```python
from build123d import *

# Parameters (mm, degrees)
SKETCH1_W                 = 38
SKETCH1_H                 = 30
BOSS_EXTRUDE1_DEPTH       = 64.4
SKETCH3_R                 = 13
BOSS_EXTRUDE3_DEPTH       = 17
SKETCH2_R                 = 4
BOSS_EXTRUDE4_DEPTH       = 18.25
SKETCH16_W                = 32
SKETCH16_H                = 58.4
CUT_EXTRUDE1_DEPTH        = 90.955669638
SKETCH17_R                = 15
BOSS_EXTRUDE9_DEPTH       = 58.4
FILLET1_R                 = 1
M3X0_5_TAPPED_HOLE1_D     = 2.5
M3X0_5_TAPPED_HOLE1_DEPTH = 3
M3X0_5_TAPPED_HOLE2_D     = 2.5
M3X0_5_TAPPED_HOLE2_DEPTH = 3
SKETCH22_R                = 4
SKETCH22_R_2              = 2.5
CUT_EXTRUDE2_DEPTH        = 13.25
FILLET2_R                 = 0.5


with BuildPart() as part:
    # Sketch1 → Boss-Extrude1 (new body)
    with BuildSketch(Plane.XY):
        Rectangle(SKETCH1_W, SKETCH1_H)
    extrude(amount=BOSS_EXTRUDE1_DEPTH)

    # Sketch3 → Boss-Extrude3 (add)
    with BuildSketch(Plane(origin=(0, 0, 0), x_dir=(-1, 0, 0), z_dir=(0, 0, -1))):
        Circle(SKETCH3_R)
    extrude(amount=BOSS_EXTRUDE3_DEPTH)

    # Sketch2 → Boss-Extrude4 (add)
    with BuildSketch(Plane.XY.offset(64.4)):
        with Locations(Location((0, 0, 0), (0, 0, 180))):
            Circle(SKETCH2_R)
    extrude(amount=BOSS_EXTRUDE4_DEPTH)

    # Sketch16 → Cut-Extrude1 (cut, through all)
    with BuildSketch(Plane.XZ.offset(15)):
        with Locations((0, 32.2)):
            Rectangle(SKETCH16_W, SKETCH16_H)
    extrude(amount=-CUT_EXTRUDE1_DEPTH, mode=Mode.SUBTRACT)

    # Sketch17 → Boss-Extrude9 (add)
    with BuildSketch(Plane(origin=(0, 0, 61.4), x_dir=(-1, 0, 0), z_dir=(0, 0, -1))):
        with Locations(Location((0, 0, 0), (0, 0, 270))):
            Circle(SKETCH17_R)
    extrude(amount=BOSS_EXTRUDE9_DEPTH)

    # Fillet1
    fillet1_edges = [part.edges().sort_by_distance(p)[0] for p in [
        (-19, 0, 64.4),
        (19, 0, 64.4),
    ]]
    fillet(fillet1_edges, radius=FILLET1_R)

    # M3x0.5 Tapped Hole1
    with Locations(Plane.ZY.offset(19)):
        with Locations((14.4, -10), (44.4, -10), (44.4, 10), (14.4, 10)):
            Hole(M3X0_5_TAPPED_HOLE1_D / 2, depth=M3X0_5_TAPPED_HOLE1_DEPTH)

    # M3x0.5 Tapped Hole2
    with Locations(Plane(origin=(19, 0, 0), x_dir=(0, 0, -1), z_dir=(1, 0, 0))):
        with Locations((-14.4, 10), (-14.4, -10), (-44.4, -10), (-44.4, 10)):
            Hole(M3X0_5_TAPPED_HOLE2_D / 2, depth=M3X0_5_TAPPED_HOLE2_DEPTH)

    # Sketch22 → Cut-Extrude2 (cut)
    with BuildSketch(Plane.XY.offset(64.4)):
        Circle(SKETCH22_R)
        Circle(SKETCH22_R_2, mode=Mode.SUBTRACT)
    extrude(amount=CUT_EXTRUDE2_DEPTH, mode=Mode.SUBTRACT)

    # Fillet2
    fillet2_edges = [part.edges().sort_by_distance(p)[0] for p in [
        (4, 0, 82.65),
    ]]
    fillet(fillet2_edges, radius=FILLET2_R)


solid = part.part
```
Read the model definition and answer for the solid it produces. Units are mm, in the model's axes. A direction names the side the tool comes from. Give positions to 0.01 mm unless a question says otherwise; leave off trailing zeros. Write each loop counter-clockwise with the first axis right and the second up, starting at its lowest first coordinate (ties: lowest second). Pieces come first, ordered by that corner, then holes. Notation, with made-up numbers: (7.5, 44.25) - (61.5, 44.25) arc R14 cw to (61.5, 49.25) - close; hole circle Ø11 at (-15.75, 76.5). An arc over 180 degrees is marked (long way). Write item = value, one per line. Start each with the question number.
Item 1: Each of these flat-tipped pins is pushed along its axis until it touches: P1, Ø1.5, axis at y = -10, z = 14.4, coming from the -X side; P2, Ø5, axis at x = -7, y = 7, coming from the +Z side; P3, Ø1.5, axis at y = -10, z = 44.4, coming from the +X side. Where does it stop, or does it pass through?
Item 2: Find section C-C (y = 0). Give the vertices of the cut face in (x, z), then the cut area to 3 significant figures.
Item 3: A tool of negligible diameter and unlimited length cuts with its end or side. For faces 4 (the cylindrical face through (17.48, -9.62, 45.59)), 5 (the flat face through (16, 0, 32)), 6 (the cylindrical face through (-17.479, -8.946, 43.728)), 7 (the flat face through (15.7, -2.3, 61.4)), from which of +Z, -Z, +X, -X, +Y, -Y can it reach the whole face along a straight path? Write none if from no direction.
Item 4: Find section B-B (z = 33.5). Give the vertices of the cut face in (x, y).
Item 5: Find section A-A (z = 44.4). Give the vertices of the cut face in (x, y), then the cut area to 3 significant figures.
Item 6: Find the intervals of material crossed by probe 1 along Z at (x, y) = (-14, 7.75); probe 2 along X at (y, z) = (13, 44); probe 3 along Y at (x, z) = (17, 44), in increasing order. Write a range as [from, to].
Item 7: Find section D-D (y = -10). State how many separate pieces and enclosed holes the cut face has, then the cut area to 3 significant figures.
Item 8: The mould has two halves that part along Y. Classify faces 1 (the flat face through (0, 0, 82.65)), 2 (the cylindrical face through (-0.66, 14.985, 32.609)), 3 (the cylindrical face through (-17.479, 11.054, 43.728)): +Y half, -Y half, draft (parallel to the pull), parting line (faces both ways), or undercut.
Response:
q1.P1 = -11.81
q1.P2 = 64.4
q1.P3 = 11.81
q2.outline = (-19, 0) - (-13, 0) - (-13, -17) - (13, -17) - (13, 0) - (19, 0) - (19, 63.4) arc R1 ccw to (18, 64.4) - (2.5, 64.4) - (2.5, 77.65) - (4, 77.65) - (4, 82.15) arc R0.5 ccw to (3.5, 82.65) - (-3.5, 82.65) arc R0.5 ccw to (-4, 82.15) - (-4, 77.65) - (-2.5, 77.65) - (-2.5, 64.4) - (-18, 64.4) arc R1 ccw to (-19, 63.4) - close; hole (-16, 3) - (-15, 3) - (-15, 61.4) - (-16, 61.4) - close; hole (15, 3) - (16, 3) - (16, 61.4) - (15, 61.4) - close
q2.area = 2,880 mm²
q3.face_4 = +X
q3.face_5 = +Y, -Y
q3.face_6 = -X
q3.face_7 = none
q4.outline = (-19, -15) - (-16, -15) - (-16, 15) - (-19, 15) - close; circle Ø30 at (0, 0); (16, -15) - (19, -15) - (19, 15) - (16, 15) - close
q5.outline = (-19, -15) - (-16, -15) - (-16, -11.25) - (-19, -11.25) - close; (-19, -8.75) - (-16, -8.75) - (-16, 8.75) - (-19, 8.75) - close; (-19, 11.25) - (-16, 11.25) - (-16, 15) - (-19, 15) - close; circle Ø30 at (0, 0); (16, -15) - (19, -15) - (19, -11.25) - (16, -11.25) - close; (16, -8.75) - (19, -8.75) - (19, 8.75) - (16, 8.75) - close; (16, 11.25) - (19, 11.25) - (19, 15) - (16, 15) - close
q5.area = 857 mm²
q6.probe_1 = [0, 3], [61.4, 64.4]
q6.probe_2 = [-19, -16], [-7.48, 7.48], [16, 19]
q6.probe_3 = [-15, -11.18], [-8.82, 8.82], [11.18, 15]
q7.separate_pieces = 3
q7.enclosed_holes = 0
q7.area = 2,140 mm²
q8.face_1 = draft
q8.face_2 = parting line
q8.face_3 = undercut
